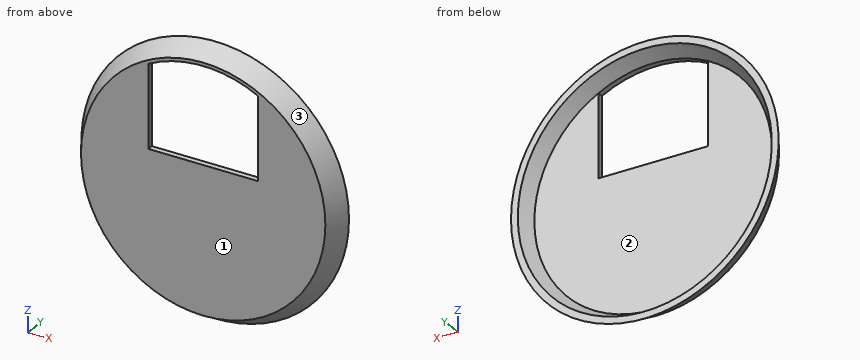
from build123d import *

# Parameters (mm, degrees)
CUT_EXTRUDE1_DEPTH = 4


with BuildPart() as part:
    # Sketch1 → Revolve1 (revolve)
    with BuildSketch(Plane.XY):
        Polygon((0, 0), (63, 0), (69, 10), (65.501428863, 10), (61.301428863, 3), (0, 3), align=None)
    revolve(axis=Axis((0, 0, 0), (0, 1, 0)))

    # Sketch2 → Cut-Extrude1 (cut, through all)
    with BuildSketch(Plane(origin=(0, 3, 0), x_dir=(1, 0, 0), z_dir=(0, 1, 0))):
        with BuildLine():
            Line((-28.3, -12), (-28.3, -54.378076287))
            ThreePointArc((-28.3, -54.378076287), (0, -61.301428863), (28.3, -54.378076287))
            Line((28.3, -54.378076287), (28.3, -12))
            Line((28.3, -12), (-28.3, -12))
        make_face()
    extrude(amount=-CUT_EXTRUDE1_DEPTH, mode=Mode.SUBTRACT)


solid = part.part
Can you work these out from the model? Positions are in its coordinate system, mm. Face numbers are marked on the shaded views. Round coordinates to 2 decimals unless told otherwise and drop trailing zeros. Order: outer loops, then holes, each group sorted by start corner. A loop starts at its lowest first (then second) coordinate and runs counter-clockwise, first axis right, second up. Notation, with made-up numbers: (61, -16) - (119, -16) arc R25 cw to (119, 16) - close; hole circle Ø3 at (14, -40). An arc over 180 degrees is marked (long way). Answer in a Markdown table with one row per item.
(1) Suppose I cut it at C-C, the plane y = 5. Please give me the cut outline in (x, z), plus the area to 3 significant figures.
From the geometry:
| item | result |
|---|---|
| outline | circle Ø132 at (0, 0); hole circle Ø125 at (0, 0) |
| area | 1,410 mm2 |
(2) Suppose I cut it at A-A, the plane x = 0. Please give me the cut outline in (y, z).
From the geometry:
| item | result |
|---|---|
| outline | (0, -63) - (10, -69) - (10, -65.5) - (3, -61.3) - (3, 12) - (0, 12) - close; (0, 61.3) - (3, 61.3) - (10, 65.5) - (10, 69) - (0, 63) - close |
(3) For P1, Ø5, axis at x = -25.5, y = 2, coming from the -Z side; P2, Ø6, axis at x = 18.5, y = 1.5, coming from the -Z side; P3, Ø0.9, axis at x = -2, y = 1.5, coming from the +Z side, each with a flat end and sliding along its axis, tell me the tip position at first contact or that it passes through.
From the geometry:
| item | result |
|---|---|
| P1 | stops at z = -60.85 |
| P2 | stops at z = -63.23 |
| P3 | stops at z = 64.14 |
(4) Please list where these lines run through material, in increasing order: L1, parallel to Y at x = -19, z = -6; L2, parallel to X at y = 2.5, z = 17; L3, parallel to X at y = 8.5, z = -32. Write a range as from..to.
From the geometry:
| item | result |
|---|---|
| L1 | y = 0..3 |
| L2 | x = -62.22..-28.3, 28.3..62.22 |
| L3 | x = -60.11..-56.12, 56.12..60.11 |
(5) If we mould it in two halves opening along Z, with no side actions, what happens to the marked faces 1, 2 and 3? For each: released by +Z, released by -Z, zero draft, split by the parting line, or undercut.
From the geometry:
| item | result |
|---|---|
| face 1 | zero draft |
| face 2 | undercut |
| face 3 | split by the parting line |
(6) Suppose I cut it at B-B, the plane z = 0. Please give me the cut outline in (x, y).
From the geometry:
| item | result |
|---|---|
| outline | (-69, 10) - (-63, 0) - (63, 0) - (69, 10) - (65.5, 10) - (61.3, 3) - (-61.3, 3) - (-65.5, 10) - close |
